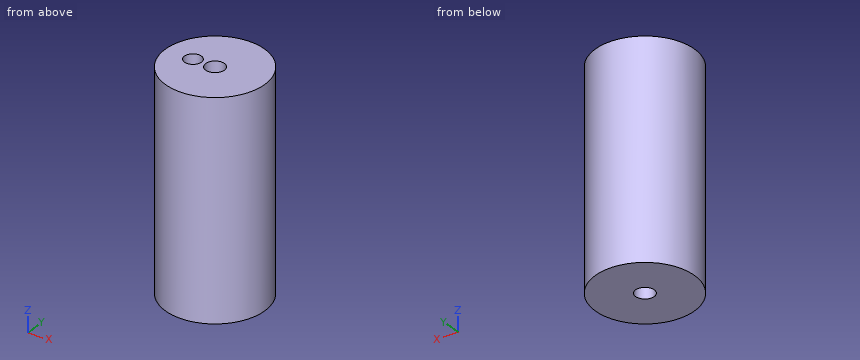
from build123d import *

# Parameters (mm, degrees)
F0_R     = 9.25
F0_R_2   = 1.75
F1_DEPTH = 25
F2_DEPTH = 15
F4_R     = 1.5899779652
F5_DEPTH = 25


with BuildPart() as f1:
    # F0 (on Top) → F1 (new body)
    with BuildSketch(Plane.XY):
        Circle(F0_R)
        Circle(F0_R_2, mode=Mode.SUBTRACT)
    extrude(amount=F1_DEPTH)

    # F2 (add): a face of the model
    f2_faces = [f1.faces().sort_by_distance(p)[0] for p in [
        (-8.988370491, 0, 0),
    ]]
    extrude(f2_faces, amount=F2_DEPTH)

    # F4 (on face) → F5 (cut)
    with BuildSketch(Plane.XY.offset(25)):
        with Locations((-4.0855864063, 0)):
            Circle(F4_R)
    extrude(amount=-F5_DEPTH, mode=Mode.SUBTRACT)


solid = f1.part
Can you work these out from the model? Positions are in its coordinate system, mm. Coordinates: 2 decimals unless noted, no trailing zeros. Loops run counter-clockwise (first coordinate to the right, second up) from the corner with the lowest first, then second, coordinate; pieces in that order, holes last. Notation, with made-up numbers: (1, 54) - (49, 54) arc R8 ccw to (49, 63) - close; hole circle Ø1 at (32, -4). An arc over 180 degrees is marked (long way). Answer as a JSON object with one key per item and string values. Group by question number.
Item 1: If we section it at D-D (z = 2.5): List the corners of the cut face in (x, y) for me, plus the area to 3 significant figures.
Item 2: If we section it at B-B (x = 0): List the corners of the cut face in (y, z) for me, plus the area to 3 significant figures.
Item 3: If we section it at A-A (y = 0): List the corners of the cut face in (x, z) for me, plus the area to 4 significant figures.
Item 4: If I drill on L1, parallel to Y at x = 0, z = -6.75; L2, parallel to X at y = 6.5, z = -12.5; L3, parallel to Y at x = -1, z = 19, over which ranges is the centre line in solid material (lowest first)? Write a range as from..to.
Item 5: If we section it at C-C (z = -9.5): List the corners of the cut face in (x, y) for me, plus the area to 3 significant figures.
Item 6: For pin 1 (5 mm diameter, centred on y = 7, z = 10.5, fed in from +X), with a flat end and sliding along its axis, tell me the tip position at first contact or that it passes through.
Returned:
{
 "1": {"outline": "circle Ø18.5 at (0, 0); hole circle Ø3.18 at (-4.09, 0); hole circle Ø3.5 at (0, 0)", "area": "251 mm²"},
 "2": {"outline": "(-9.25, -15) - (-1.75, -15) - (-1.75, 25) - (-9.25, 25) - close; (1.75, -15) - (9.25, -15) - (9.25, 25) - (1.75, 25) - close", "area": "600 mm²"},
 "3": {"outline": "(-9.25, -15) - (-1.75, -15) - (-1.75, 25) - (-2.5, 25) - (-2.5, 0) - (-5.68, 0) - (-5.68, 25) - (-9.25, 25) - close; (1.75, -15) - (9.25, -15) - (9.25, 25) - (1.75, 25) - close", "area": "520.5 mm²"},
 "4": {"L1": "y = -9.25..-1.75, 1.75..9.25", "L2": "x = -6.58..6.58", "L3": "y = -9.2..-1.44, 1.44..9.2"},
 "5": {"outline": "circle Ø18.5 at (0, 0); hole circle Ø3.5 at (0, 0)", "area": "259 mm²"},
 "6": {"pin 1": "stops at x = 8.08"}
}
